```python
from build123d import *

# Parameters (mm, degrees)
EXTRUDE_1_DEPTH = 820


with BuildPart() as part:
    # Эскиз1 → Бобышка-Вытянуть1 (new body)
    with BuildSketch(Plane.XY):
        Polygon((0, 0), (0, 170), (35, 170), (35, 0), (25, 0), (25, 15), (10, 15), (10, 0), align=None)
    extrude(amount=-EXTRUDE_1_DEPTH)


solid = part.part
```
The listing builds one solid part. Answer for the finished solid, in the listing's coordinates (mm). A direction names the side the tool comes from. Round coordinates to 2 decimals unless told otherwise and drop trailing zeros. Order: outer loops, then holes, each group sorted by start corner. A loop starts at its lowest first (then second) coordinate and runs counter-clockwise, first axis right, second up. Notation, with made-up numbers: (27, 40) -> (38, 40) arc R26 cw to (38, 67) -> close; hole circle Ø7 at (73, 0). An arc over 180 degrees is marked (long way). Answer as CSV lines item,"result".
Q1. Consider line 1 (Y direction, x = 14.5, z = -525.5). Determine where the line is inside the solid, lowest interval first. Write a range as from..to.
Computed values:
line 1,"y = 15..170"
Q2. A cutting plane is placed at A-A on z = -536.5. Determine the outline of the cut face in (x, y).
Computed values:
outline,"(0, 0) -> (10, 0) -> (10, 15) -> (25, 15) -> (25, 0) -> (35, 0) -> (35, 170) -> (0, 170) -> close"
Q3. Which of the six approach directions +Z, -Z, +X, -X, +Y, -Y give full straight-line access (tool end or side, diameter ignored) to faces 1 (the flat face through (25, 7, -404)), 2 (the flat face through (18, 86, -820))?
Computed values:
face 1,"+Z, -Z, -Y"
face 2,"-Z, +X, -X, +Y, -Y"
Q4. For a pull along X with two mould halves and no side action, classify faces 3 (the flat face through (0, 84, -404)), 4 (the flat face through (10, 8, -404)), 5 (the flat face through (18, 86, 0)) as +X half, -X half, draft (parallel to the pull), parting line (faces both ways), or undercut.
Computed values:
face 3,"-X half"
face 4,"undercut"
face 5,"draft"
Q5. Given pin 1 (5 mm diameter, centred on x = 29.5, y = 61, fed in from +Z); pin 2 (7.5 mm diameter, centred on x = 17.5, z = -504, fed in from -Y), each flat-ended and moving along its own axis, determine where each tip first touches the part or whether it passes through.
Computed values:
pin 1,"stops at z = 0"
pin 2,"stops at y = 15"
